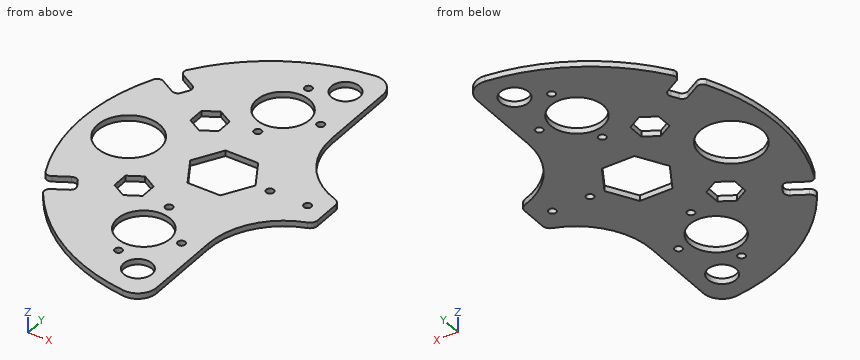
```python
from build123d import *

# Parameters (mm, degrees)
SKETCH_2_R             = 2
SKETCH_2_R_2           = 14
SKETCH_2_R_3           = 16.5
SKETCH_2_W             = 30
SKETCH_2_H             = 20
EXTRUDE_1_DEPTH        = 3
FILLET_1_R             = 40
FILLET_2_R             = 10
SKETCH_3_R             = 7.5
CUT_EXTRUDE_1_DEPTH    = 142.05975465
FILLET_3_R             = 3
FILLET_3_OF_MIRROR_1_R = 3
SKETCH_4_R             = 2
CUT_EXTRUDE_2_DEPTH    = 142.05975465
FILLET_4_R             = 4


with BuildPart() as part:
    # 草图2 → 凸台-拉伸1 (new body)
    # profile 1 of 2: a face of its own
    with BuildSketch(Plane.XY):
        with BuildLine():
            Line((0, 10), (0, 100))
            ThreePointArc((0, 100), (-100, 0), (0, -100))
            Line((0, -100), (0, -10))
            Line((0, -10), (0, 10))
        make_face()
        with Locations((-30, -75)):
            Circle(SKETCH_2_R, mode=Mode.SUBTRACT)
        with Locations((-30, -55)):
            Circle(SKETCH_2_R_2, mode=Mode.SUBTRACT)
        with Locations((-10, -55)):
            Circle(SKETCH_2_R, mode=Mode.SUBTRACT)
        with Locations((-30, -35)):
            Circle(SKETCH_2_R, mode=Mode.SUBTRACT)
        with Locations((-75, 0)):
            Circle(SKETCH_2_R_3, mode=Mode.SUBTRACT)
        with Locations((-30, 35)):
            Circle(SKETCH_2_R, mode=Mode.SUBTRACT)
        with Locations((-30, 55)):
            Circle(SKETCH_2_R_2, mode=Mode.SUBTRACT)
        with Locations((-10, 55)):
            Circle(SKETCH_2_R, mode=Mode.SUBTRACT)
        with Locations((-30, 75)):
            Circle(SKETCH_2_R, mode=Mode.SUBTRACT)
    # profile 2 of 2: a face of its own
    with BuildSketch(Plane.XY):
        with Locations((15, 0)):
            Rectangle(SKETCH_2_W, SKETCH_2_H)
    extrude(amount=EXTRUDE_1_DEPTH)

    # 圆角1
    # the kernel refuses this fillet: 40 mm, written as the material it adds along each edge
    with BuildSketch(Plane(origin=(0, 10, 0), x_dir=(0, 1, 0), z_dir=(0, 0, 1))) as fillet_1_piece_1:
        with BuildLine():
            CenterArc((38.729833462, -40), FILLET_1_R, 90, 75.522487814)
            Line((0, -30), (-0.774596669, -29.8))
            ThreePointArc((-0.774596669, -29.8), (-0.8, -15), (-0.8, 0))
            Line((-0.8, 0), (0, 0.8))
            Line((0, 0.8), (38.729833462, 0.8))
            Line((38.729833462, 0.8), (38.729833462, 0))
        make_face()
    extrude(amount=3)
    with BuildSketch(Plane(origin=(0, -10, 0), x_dir=(0, -1, 0), z_dir=(0, 0, 1))) as fillet_1_piece_2:
        with BuildLine():
            CenterArc((38.729833462, 40), FILLET_1_R, 194.477512186, 75.522487814)
            Line((0, 30), (-0.774596669, 29.8))
            ThreePointArc((-0.774596669, 29.8), (-0.8, 15), (-0.8, 0))
            Line((-0.8, 0), (0, -0.8))
            Line((0, -0.8), (38.729833462, -0.8))
            Line((38.729833462, -0.8), (38.729833462, 0))
        make_face()
    extrude(amount=3)

    # 圆角2
    fillet_2_edges = [part.edges().sort_by_distance(p)[0] for p in [
        (0, 100, 1.5),
        (0, -100, 1.5),
    ]]
    fillet(fillet_2_edges, radius=FILLET_2_R)

    # 草图3 → 切除-拉伸1 (cut, through all)
    with BuildSketch(Plane.XY.offset(3)):
        with BuildLine():
            Line((-76.112159322, 38.169872981), (-71.112159322, 46.830127019))
            Line((-71.112159322, 46.830127019), (-83.99421946, 54.267587908))
            ThreePointArc((-83.99421946, 54.267587908), (-86.602540378, 50), (-88.99421946, 45.60733387))
            Line((-88.99421946, 45.60733387), (-76.112159322, 38.169872981))
        make_face()
        Polygon((-42.320508076, 0), (-33.660254038, -15), (-16.339745962, -15), (-7.679491924, 0), (-16.339745962, 15), (-33.660254038, 15), align=None)
        Polygon((-59.461524227, 34.330127019), (-59.461524227, 25.669872981), (-51.961524227, 21.339745962), (-44.461524227, 25.669872981), (-44.461524227, 34.330127019), (-51.961524227, 38.660254038), align=None)
        with Locations((-15, 82)):
            Circle(SKETCH_3_R)
    cut_extrude_1 = extrude(amount=-CUT_EXTRUDE_1_DEPTH, mode=Mode.SUBTRACT)

    # 圆角3
    fillet_3_edges = [part.edges().sort_by_distance(p)[0] for p in [
        (-71.112159322, 46.830127019, 1.5),
        (-76.112159322, 38.169872981, 1.5),
        (-88.99421946, 45.60733387, 1.5),
        (-83.99421946, 54.267587908, 1.5),
    ]]
    fillet(fillet_3_edges, radius=FILLET_3_R)

    # 镜向1: 切除-拉伸1 across plane
    add(cut_extrude_1.mirror(Plane.ZX), mode=Mode.SUBTRACT)

    # 圆角3 of 镜向1
    fillet_3_of_mirror_1_edges = [part.edges().sort_by_distance(p)[0] for p in [
        (-71.112159322, -46.830127019, 1.5),
        (-76.112159322, -38.169872981, 1.5),
        (-88.99421946, -45.60733387, 1.5),
        (-83.99421946, -54.267587908, 1.5),
    ]]
    fillet(fillet_3_of_mirror_1_edges, radius=FILLET_3_OF_MIRROR_1_R)

    # 草图4 → 切除-拉伸2 (cut, through all)
    with BuildSketch(Plane.XY.offset(3)):
        with Locations((20, 0)):
            Circle(SKETCH_4_R)
        Circle(SKETCH_4_R)
    extrude(amount=-CUT_EXTRUDE_2_DEPTH, mode=Mode.SUBTRACT)

    # 圆角4
    fillet_4_edges = [part.edges().sort_by_distance(p)[0] for p in [
        (30, 10, 1.5),
        (30, -10, 1.5),
    ]]
    fillet(fillet_4_edges, radius=FILLET_4_R)


solid = part.part
```
The listing builds one solid part. Answer for the finished solid, in the listing's coordinates (mm). Coordinates: 2 decimals unless noted, no trailing zeros. Loops run counter-clockwise (first coordinate to the right, second up) from the corner with the lowest first, then second, coordinate; pieces in that order, holes last. Notation, with made-up numbers: (3, 12) -> (55, 12) arc R16 cw to (55, 43) -> close; hole circle Ø10 at (45.5, -9.5). An arc over 180 degrees is marked (long way). Return JSON: item names as keys, results as strings. Group by question number.
(1) A cutting plane is placed at A-A on y = -86.5. Write down the section's boundary in (x, z), and give its area (3 significant figures).
(2) Given pin 1 Ø5 at (x, y) = (14.5, 17) entering from -Z; pin 2 Ø1 at (y, z) = (-51.5, 1.5) entering from -X; pin 3 Ø1 at (y, z) = (-29.5, 0.5) entering from -X; pin 4 Ø0.9 at (x, z) = (-23.5, 2) entering from +Y, each flat-ended and moving along its own axis, determine where each tip first touches the part or whether it passes through.
(3) A cutting plane is placed at D-D on z = 0.55. Count the separate pieces of the cut face and the enclosed holes in it, and give its area (3 significant figures).
(4) A cutting plane is placed at B-B on y = 55. Write down the section's boundary in (x, z).
(5) A cutting plane is placed at C-C on x = -63. Write down the section's boundary in (y, z), and give its area (3 significant figures).
(6) Find the intervals of material crossed by probe 1 along Y at (x, z) = (-39, 2.05); probe 2 along Y at (x, z) = (-10, 0.95); probe 3 along Y at (x, z) = (-47, 0.9), in increasing order. Write a range as from..to.
The answers:
{
 "1": {"outline": "(-50.18, 0) -> (-21, 0) -> (-21, 3) -> (-50.18, 3) -> close; (-9, 0) -> (0, 0) -> (0, 3) -> (-9, 3) -> close", "area": "115 mm^2"},
 "2": {"pin 1": "stops at z = 0", "pin 2": "stops at x = -80.07", "pin 3": "stops at x = -95.7", "pin 4": "stops at y = 97.31"},
 "3": {"separate pieces": "1", "enclosed holes": "16", "area": "12,800 mm^2"},
 "4": {"outline": "(-82.71, 0) -> (-44, 0) -> (-44, 3) -> (-82.71, 3) -> close; (-16, 0) -> (-12, 0) -> (-12, 3) -> (-16, 3) -> close; (-8, 0) -> (0, 0) -> (0, 3) -> (-8, 3) -> close"},
 "5": {"outline": "(-77.66, 0) -> (-11.32, 0) -> (-11.32, 3) -> (-77.66, 3) -> close; (11.32, 0) -> (77.66, 0) -> (77.66, 3) -> (11.32, 3) -> close", "area": "398 mm^2"},
 "6": {"probe 1": "y = -92.08..-65.72, -44.28..-5.75, 5.75..44.28, 65.72..92.08", "probe 2": "y = -99.44..-87.59, -76.41..-57, -53..-4.02, 4.02..53, 57..76.41, 87.59..99.44", "probe 3": "y = -88.27..-35.8, -24.2..24.2, 35.8..88.27"}
}
